Input: dimensioned drawing with shaded views. Units: mm. Origin: part minimum x, y, z. Coordinates: 2 decimals unless noted, no trailing zeros. Loops run counter-clockwise (first coordinate to the right, second up) from the corner with the lowest first, then second, coordinate; pieces in that order, holes last. Notation, with made-up numbers: (11, -15.75) -> (54, -15.75) arc R36 cw to (54, 19.25) -> close; hole circle Ø4 at (21, 55). An arc over 180 degrees is marked (long way). Answer as CSV lines item,"result".
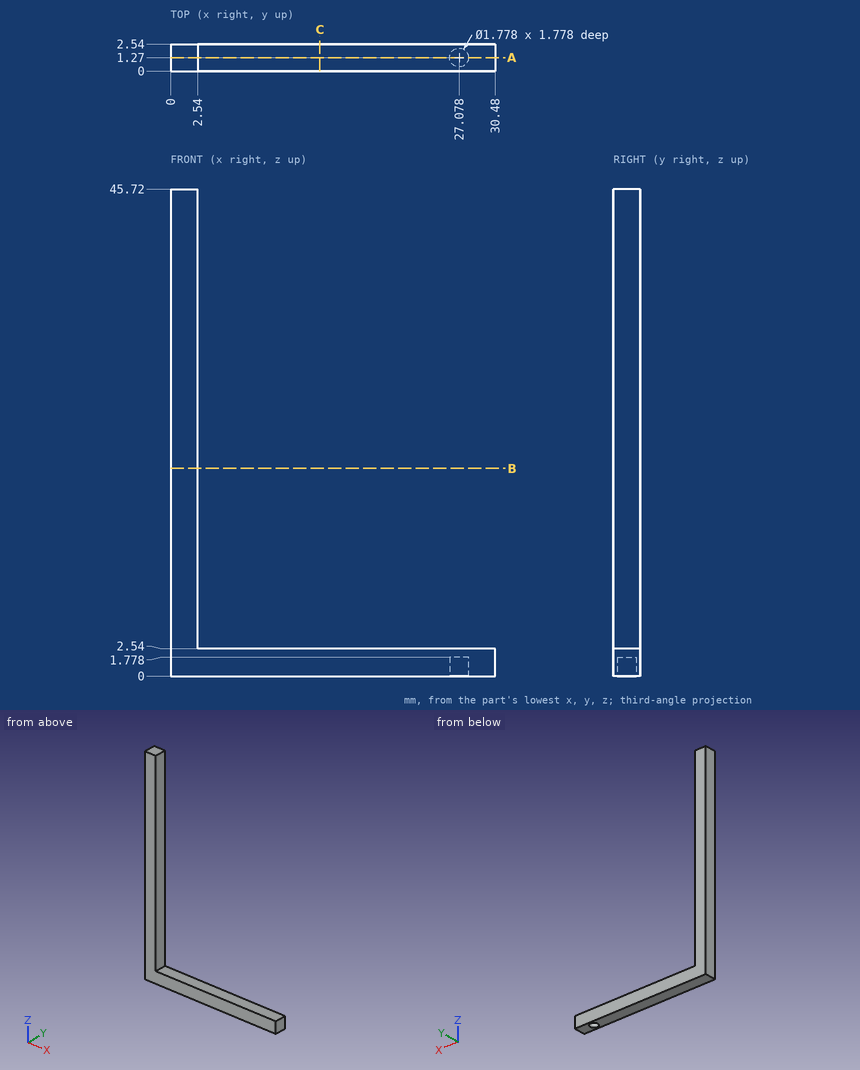
(1) Cut plane B-B (z = 19.5). Return the cut outline in (x, y).
Computed values:
outline,"(0, 0) -> (2.54, 0) -> (2.54, 2.54) -> (0, 2.54) -> close"
(2) Material intervals for L1, parallel to X at y = 1.2, z = 17, sorted ascending. Write a range as [from, to].
Computed values:
L1,"[0, 2.54]"
(3) Cut plane A-A (y = 1.27). Return the cut outline in (x, z).
Computed values:
outline,"(0, 0) -> (26.19, 0) -> (26.19, 1.78) -> (27.97, 1.78) -> (27.97, 0) -> (30.48, 0) -> (30.48, 2.54) -> (2.54, 2.54) -> (2.54, 45.72) -> (0, 45.72) -> close"
(4) Pin query (flat end, axial travel): pin 1 Ø1.3 at (x, y) = (23, 1.5) entering from +Z; pin 2 Ø0.8 at (y, z) = (1, 34) entering from +X. Return the tip coordinate at first contact, or that it passes through.
Computed values:
pin 1,"z = 2.54"
pin 2,"x = 2.54"
